Input: dimensioned drawing with shaded views. Units: mm. Origin: part minimum x, y, z. A direction names the side the tool comes from. Coordinates: 2 decimals unless noted, no trailing zeros. Write each loop counter-clockwise with the first axis right and the second up, starting at its lowest first coordinate (ties: lowest second). Pieces come first, ordered by that corner, then holes. Notation, with made-up numbers: (-2.5, 49) -> (18.5, 49) arc R8 cw to (18.5, 63) -> close; hole circle Ø2 at (24.25, 89.25). An arc over 180 degrees is marked (long way). One line per item, written item: value. Start each with the question number.
1. Line query: line 1 (X direction, y = 11.2, z = 35); line 2 (X direction, y = 9.5, z = 37); line 3 (Y direction, x = 3, z = 7). Output: solid intervals per line, ascending.
2. First-contact query: P1, Ø3, axis at x = 35.5, z = 4.5, coming from the +Y side; P2, Ø11, axis at x = 22, z = 21.5, coming from the -Y side. Flat tips, straight axial feed; report the tip coordinate or a pass-through.
3. Section query A-A, the plane z = 20. Output: boundary loops of the cut face in (x, y), and give its area (3 significant figures).
4. Mould query, pull axis X, two halves, no side actions, for the marked faces 3, 4 and 5. Classes: released by +X, released by -X, zero draft, split by the parting line, or undercut.
5. Section query C-C, the plane y = 3.75. Output: boundary loops of the cut face in (x, z).
6. Access query for the marked faces 1 and 2. Directions: +Z, -Z, +X, -X, +Y, -Y. A direction counts if a zero-diameter tool reaches every point of the face in a straight line with its end or side. Return the directions, or none.
7. Section query B-B, the plane x = 35. Output: boundary loops of the cut face in (y, z), and give its area (3 significant figures).
8. Section query D-D, the plane x = 20. Output: boundary loops of the cut face in (y, z).
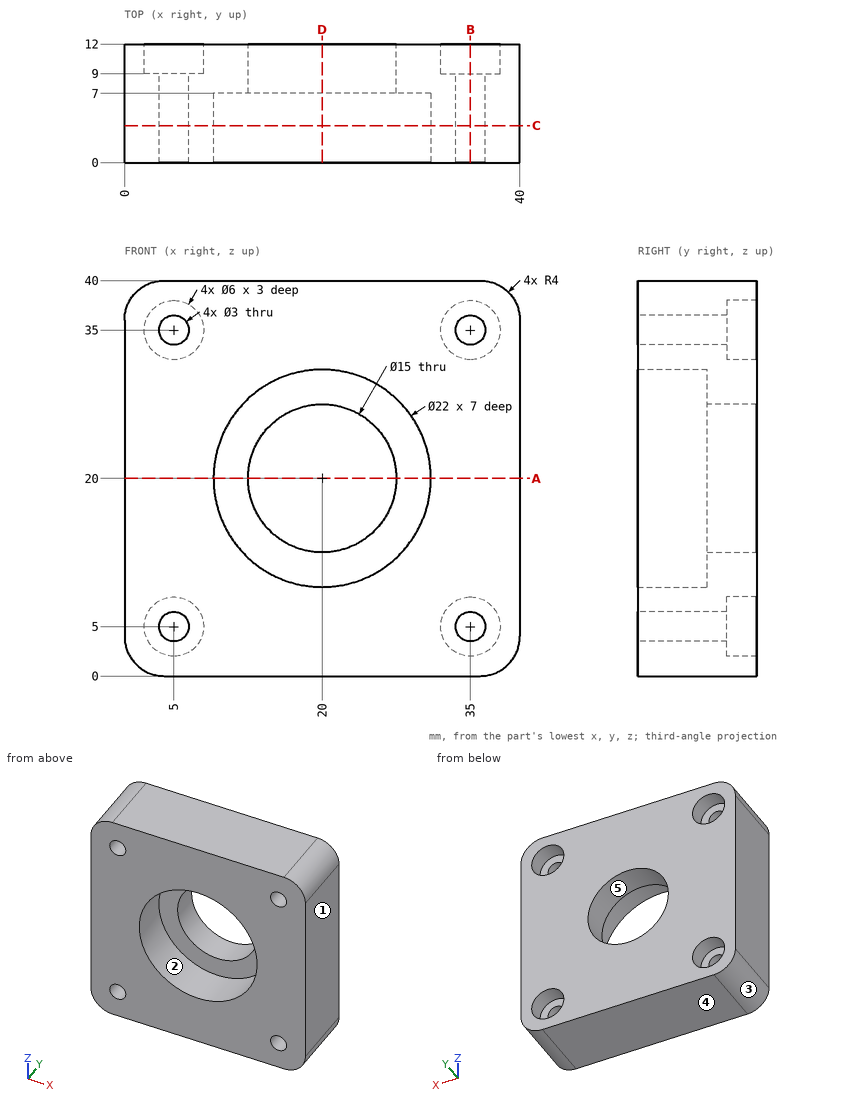
Computed values:
1. line 1: x = 0 to 2, 8 to 32, 38 to 40
1. line 2: x = 0.13 to 2.76, 7.24 to 32.76, 37.24 to 39.87
1. line 3: y = 0 to 9
2. P1: stops at y = 9
2. P2: stops at y = 7
3. outline: (0, 0) -> (9, 0) -> (9, 7) -> (12.5, 7) -> (12.5, 12) -> (0, 12) -> close; (27.5, 7) -> (31, 7) -> (31, 0) -> (40, 0) -> (40, 12) -> (27.5, 12) -> close
3. area: 251 mm²
4. face 3: released by -X
4. face 4: zero draft
4. face 5: undercut
5. outline: (0, 4) arc R4 ccw to (4, 0) -> (36, 0) arc R4 ccw to (40, 4) -> (40, 36) arc R4 ccw to (36, 40) -> (4, 40) arc R4 ccw to (0, 36) -> close; hole circle Ø3 at (5, 5); hole circle Ø3 at (5, 35); hole circle Ø22 at (20, 20); hole circle Ø3 at (35, 5); hole circle Ø3 at (35, 35)
6. face 1: +Z, -Z, +X, +Y, -Y
6. face 2: -Y
7. outline: (0, 0) -> (12, 0) -> (12, 2) -> (9, 2) -> (9, 3.5) -> (0, 3.5) -> close; (0, 6.5) -> (9, 6.5) -> (9, 8) -> (12, 8) -> (12, 32) -> (9, 32) -> (9, 33.5) -> (0, 33.5) -> close; (0, 36.5) -> (9, 36.5) -> (9, 38) -> (12, 38) -> (12, 40) -> (0, 40) -> close
7. area: 390 mm²
8. outline: (0, 0) -> (12, 0) -> (12, 12.5) -> (7, 12.5) -> (7, 9) -> (0, 9) -> close; (0, 31) -> (7, 31) -> (7, 27.5) -> (12, 27.5) -> (12, 40) -> (0, 40) -> close
